The figure shows three views and two pictorial views of one solid part (mm, origin at its lowest corner). Answer the questions. A direction names the side the tool comes from. Give positions to 0.01 mm unless a question says otherwise; leave off trailing zeros. Write each loop counter-clockwise with the first axis right and the second up, starting at its lowest first coordinate (ties: lowest second). Pieces come first, ordered by that corner, then holes. Notation, with made-up numbers: (61, -24.5) -> (83, -24.5) arc R30 cw to (83, -1.5) -> close; hole circle Ø9 at (-6, 52.5). An arc over 180 degrees is marked (long way). Answer as CSV lines item,"result". Start each with the question number.
1. Find the intervals of material crossed by line 1 (X direction, y = 10.6, z = 3); line 2 (Y direction, x = 15, z = 10.8); line 3 (X direction, y = 11.5, z = 4), in increasing order.
2. The part is cut by section B-B, the plane y = 5. Determine the outline of the cut face in (x, z), and give its area (3 significant figures).
3. A tool of negligible diameter and unlimited length cuts with its end or side. For the marked faces 5 and 6, from which of +Z, -Z, +X, -X, +Y, -Y can it reach the whole face along a straight path? Write none if from no direction.
4. The part is cut by section A-A, the plane z = 11.75. Determine the outline of the cut face in (x, y), and give its area (3 significant figures).
5. Given pin 1 (4 mm diameter, centred on x = 5, y = 5, fed in from -Z); pin 2 (4.5 mm diameter, centred on x = 14.8, z = 3, fed in from -Y); pin 3 (4 mm diameter, centred on x = 12, z = 8, fed in from -Y); pin 4 (5.5 mm diameter, centred on x = 9, y = 5, fed in from -Z), each flat-ended and moving along its own axis, determine where each tip first touches the part or whether it passes through.
6. The part is cut by section C-C, the plane y = 11. Determine the outline of the cut face in (x, z).
7. For a pull along X with two mould halves and no side action, classify the marked faces 1, 2, 3 and 4 as pulls with the +X half, pulls with the -X half, needs draft (parallel to the pull), parting line crosses it, or undercut.
8. The part is cut by section D-D, the plane x = 5.2. Determine the outline of the cut face in (y, z), and give its area (3 significant figures).
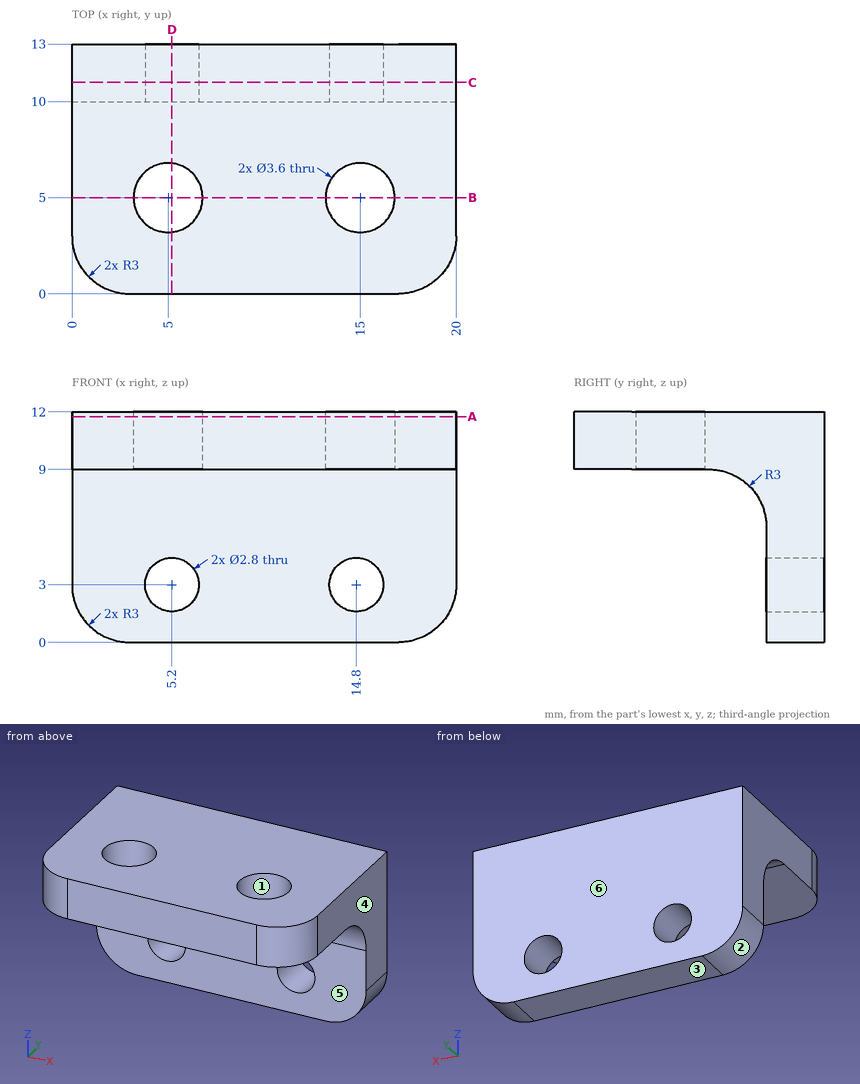
Results found:
1,line 1,"x = 0 to 3.8, 6.6 to 13.4, 16.2 to 20"
1,line 2,"y = 0 to 3.2, 6.8 to 13"
1,line 3,"x = 0 to 4.22, 6.18 to 13.82, 15.78 to 20"
2,outline,"(0, 9) -> (3.2, 9) -> (3.2, 12) -> (0, 12) -> close; (6.8, 9) -> (13.2, 9) -> (13.2, 12) -> (6.8, 12) -> close; (16.8, 9) -> (20, 9) -> (20, 12) -> (16.8, 12) -> close"
2,area,"38.4 mm²"
3,face 5,"-Z, +X, -X, -Y"
3,face 6,"+Z, -Z, +X, -X, +Y"
4,outline,"(0, 3) arc R3 ccw to (3, 0) -> (17, 0) arc R3 ccw to (20, 3) -> (20, 13) -> (0, 13) -> close; hole circle Ø3.6 at (5, 5); hole circle Ø3.6 at (15, 5)"
4,area,"236 mm²"
5,pin 1,"stops at z = 9"
5,pin 2,"stops at y = 10"
5,pin 3,"stops at y = 0"
5,pin 4,"stops at z = 8.9"
6,outline,"(0, 3) arc R3 ccw to (3, 0) -> (17, 0) arc R3 ccw to (20, 3) -> (20, 12) -> (0, 12) -> close; hole circle Ø2.8 at (5.2, 3); hole circle Ø2.8 at (14.8, 3)"
7,face 1,"undercut"
7,face 2,"pulls with the -X half"
7,face 3,"needs draft"
7,face 4,"pulls with the +X half"
8,outline,"(0, 9) -> (3.21, 9) -> (3.21, 12) -> (0, 12) -> close; (6.79, 9) -> (7, 9) arc R3 cw to (10, 6) -> (10, 4.4) -> (13, 4.4) -> (13, 12) -> (6.79, 12) -> close; (10, 0) -> (13, 0) -> (13, 1.6) -> (10, 1.6) -> close"
8,area,"48.8 mm²"
